from build123d import *

# Parameters (mm, degrees)
PAD_DEPTH    = 10
POCKET_DEPTH = 10.001


with BuildPart() as part:
    # Sketch → Pad (new body)
    with BuildSketch(Plane.YZ):
        Polygon((0, 0), (0, 240), (450, 240), (450, 0), (225, 0), align=None)
    extrude(amount=-PAD_DEPTH)

    # Sketch001 → Pocket (cut, through all)
    with BuildSketch(Plane.YZ):
        Polygon((225, 70.62109), (208.541263, 70.62109), (225, 109.167255), (241.458737, 70.62109), align=None)
    extrude(amount=-POCKET_DEPTH, mode=Mode.SUBTRACT)


solid = part.part
Here's how the part is built. I have some questions about the finished solid (model axes, mm). A direction names the side the tool comes from. Round coordinates to 2 decimals unless told otherwise and drop trailing zeros. Order: outer loops, then holes, each group sorted by start corner. A loop starts at its lowest first (then second) coordinate and runs counter-clockwise, first axis right, second up. Notation, with made-up numbers: (37.25, 51) -> (53.25, 51) arc R6 ccw to (53.25, 60) -> close; hole circle Ø9 at (5.5, 19). An arc over 180 degrees is marked (long way). Return JSON: item names as keys, results as strings.
Q1. If we mould it in two halves opening along Z, with no side actions, what happens to faces 3 (the flat face through (-5, 0, 118)), 4 (the flat face through (-4.9, 233.1, 90.2)), 5 (the flat face through (-5, 222, 0)), 6 (the flat face through (-5, 222, 240))? For each: released by +Z, released by -Z, zero draft, split by the parting line, or undercut.
Filled sheet:
{"face 3": "zero draft", "face 4": "undercut", "face 5": "released by -Z", "face 6": "released by +Z"}
Q2. If we section it at A-A on z = 76.5: List the corners of the cut face in (x, y) for me.
Filled sheet:
{"outline": "(-10, 0) -> (0, 0) -> (0, 211.05) -> (-10, 211.05) -> close; (-10, 238.95) -> (0, 238.95) -> (0, 450) -> (-10, 450) -> close"}
Q3. Which directions (+Z, -Z, +X, -X, +Y, -Y) give clear straight access to the entire face, cutting with the end or side of a thin tool? Please do faces 1 (the flat face through (0, 228, 122)), 2 (the flat face through (-5, 225, 70.621)).
Filled sheet:
{"face 1": "+Z, -Z, +X, +Y, -Y", "face 2": "+X, -X"}
Q4. I need wall thicknesses on line 1 along Y through (x, z) = (-1, 99); line 2 along Y through (x, z) = (-0.25, 78.5). Which ranges of each line are inside material? Lowest first, please. Write a range as from..to.
Filled sheet:
{"line 1": "y = 0..220.66, 229.34..450", "line 2": "y = 0..211.91, 238.09..450"}
Q5. If we section it at B-B on y = 230.5: List the corners of the cut face in (x, z) for me.
Filled sheet:
{"outline": "(-10, 0) -> (0, 0) -> (0, 70.62) -> (-10, 70.62) -> close; (-10, 96.29) -> (0, 96.29) -> (0, 240) -> (-10, 240) -> close"}
